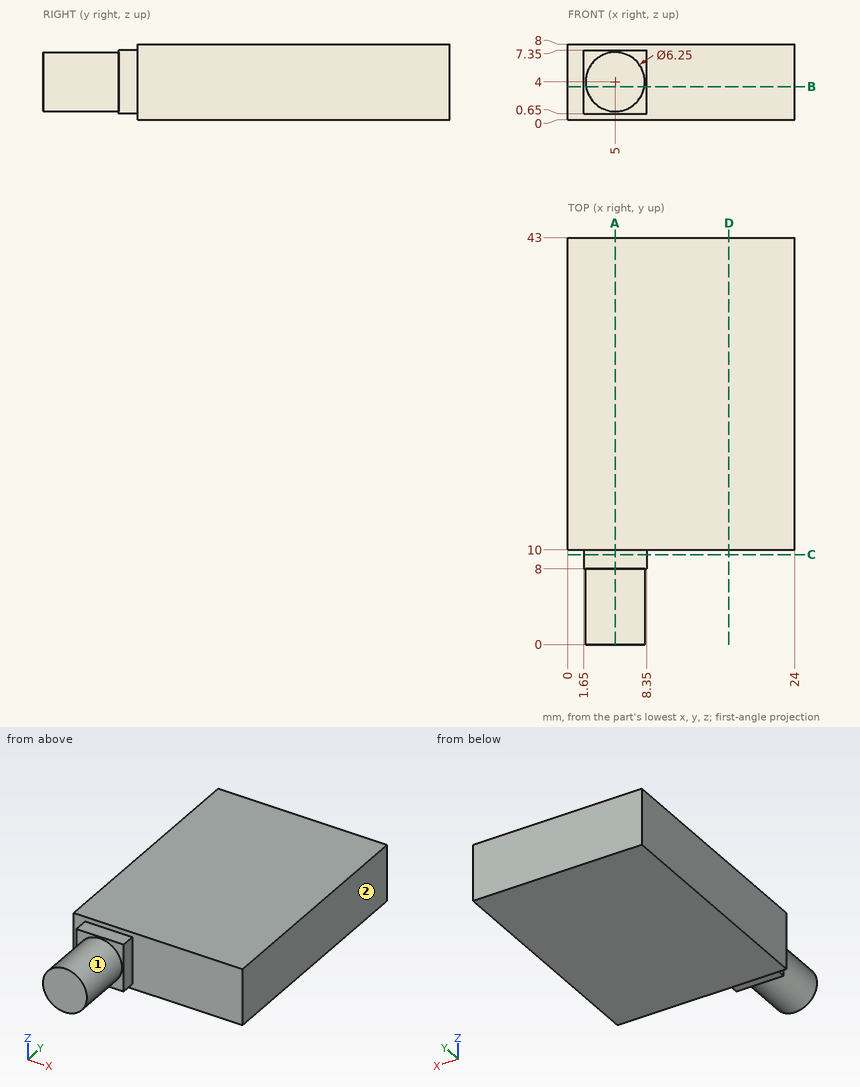
The drawing under review shows one solid part. Ordinate dimensions are in mm from its lowest x, y, z. A direction names the side the tool comes from. Round coordinates to 2 decimals unless told otherwise and drop trailing zeros. Write each loop counter-clockwise with the first axis right and the second up, starting at its lowest first coordinate (ties: lowest second). Pieces come first, ordered by that corner, then holes. Notation, with made-up numbers: (23, 39.25) - (29, 39.25) arc R11 ccw to (29, 43.25) - close; hole circle Ø2 at (19.5, 38). An arc over 180 degrees is marked (long way). Write each question's results on one line, items separated by ' | '.
Item 1: Take a section at B-B on z = 3.5. State the section outline as (x, y) points.
Calculated:
outline: (0, 10) - (1.65, 10) - (1.65, 8) - (1.92, 8) - (1.92, 0) - (8.08, 0) - (8.08, 8) - (8.35, 8) - (8.35, 10) - (24, 10) - (24, 43) - (0, 43) - close
Item 2: Take a section at D-D on x = 17. State the section outline as (y, z) points, then the cut area to 3 significant figures.
Calculated:
outline: (10, 0) - (43, 0) - (43, 8) - (10, 8) - close | area: 264 mm^2
Item 3: Take a section at C-C on y = 9.5. State the section outline as (x, z) points.
Calculated:
outline: (1.65, 0.65) - (8.35, 0.65) - (8.35, 7.35) - (1.65, 7.35) - close
Item 4: For pin 1 (1.6 mm diameter, centred on x = 4, y = 8.5, fed in from -Z); pin 2 (1 mm diameter, centred on y = 9, z = 5, fed in from +X); pin 3 (1.6 mm diameter, centred on x = 4, y = 8.5, fed in from +Z), all flat-tipped, find the tip position at first contact; note any pin that passes through.
Calculated:
pin 1: stops at z = 0.65 | pin 2: stops at x = 8.35 | pin 3: stops at z = 7.35
Item 5: To check wall thickness, follow line 1 along Y through (x, z) = (22.25, 6); line 2 along X through (y, z) = (6, 5.25); line 3 along X through (y, z) = (3.5, 3.25). State the ranges of each line that lie inside material, in increasing order. Write a range as from..to.
Calculated:
line 1: y = 10..43 | line 2: x = 2.14..7.86 | line 3: x = 1.97..8.03
Item 6: Take a section at A-A on x = 5. State the section outline as (y, z) points (3 decimals), then the cut area to 3 significant figures.
Calculated:
outline: (0, 0.875) - (8, 0.875) - (8, 0.65) - (10, 0.65) - (10, 0) - (43, 0) - (43, 8) - (10, 8) - (10, 7.35) - (8, 7.35) - (8, 7.125) - (0, 7.125) - close | area: 327 mm^2
Item 7: For the marked faces 1 and 2, list the 3-axis set-ups (+Z, -Z, +X, -X, +Y, -Y) from which the entire face can be reached by the end or side of a thin tool; tool diameter is ignored.
Calculated:
face 1: -Y | face 2: +Z, -Z, +X, +Y, -Y
